Model file for the job. Use its own axes, mm. Face numbers are marked on the shaded views. A direction names the side the tool comes from. Round coordinates to 2 decimals unless told otherwise and drop trailing zeros. Order: outer loops, then holes, each group sorted by start corner. A loop starts at its lowest first (then second) coordinate and runs counter-clockwise, first axis right, second up. Notation, with made-up numbers: (88, -15.75) -> (113, -15.75) arc R25 ccw to (113, 10.25) -> close; hole circle Ø10 at (52, 32.5). An arc over 180 degrees is marked (long way). Put each result on its own line as item: value. Start each with the question number.
Q1. Flat gauge pins, fed straight in: P1, Ø1.5, axis at x = -7.5, z = 2.5, coming from the -Y side; P2, Ø9, axis at x = 0, y = 0, coming from the +Z side; P3, Ø1.5, axis at y = 3, z = 2, coming from the +X side; P4, Ø2, axis at y = 0.5, z = 1, coming from the -X side. Where does each tip first touch, or does it go through?
Q2. Cut at B-B, the plane y = -9. List the corners of the cut face in (x, z), and give its area (3 significant figures).
Q3. Pull direction X, two halves, no side cores. Call the marked faces 5, 6 and 7: released by +X, released by -X, zero draft, split by the parting line, or undercut.
Q4. 3-axis set-ups, long thin cutter, end or side, ignore diameter. For the marked faces 1, 2, 3 and 4: which of +Z, -Z, +X, -X, +Y, -Y reach the whole face in a straight line?
Q5. Probe L1, parallel to Y at x = 0, z = 3.05; L2, parallel to Y at x = -16.5, z = 2.05; L3, parallel to Y at x = 18, z = 3.5. List the from-to ranges inside material, lowest first.
Q6. Cut at A-A, the plane x = 0. List the corners of the cut face in (y, z).
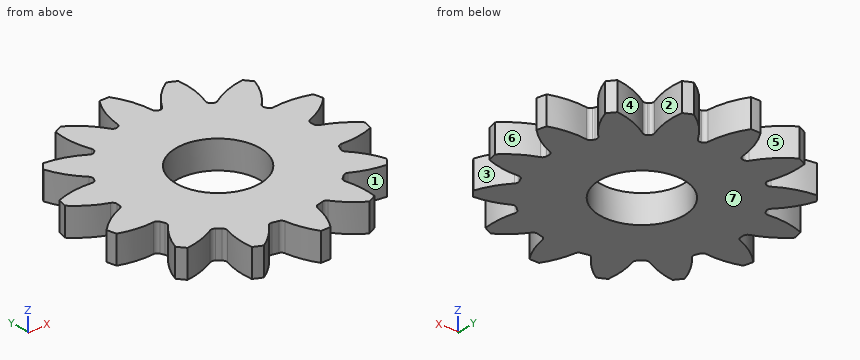
from build123d import *

# Parameters (mm, degrees)
SKETCH_1_R               = 17.25
EXTRUDE_1_DEPTH          = 5
EXTRUDE_2_DEPTH          = 5
FILLET_1_R               = 0.75
PATTERN_CIRCULAR_1_DEPTH = 5
CUT_EXTRUDE_2_REACH      = 35.573
SKETCH_2_R               = 7.5


# Read off the part's stored shape, not the designer's step: 원형 패턴1
with BuildPart() as part:
    # 스케치1 → 보스-돌출1 (new body)
    with BuildSketch(Plane.XY):
        Circle(SKETCH_1_R)
    extrude(amount=EXTRUDE_1_DEPTH)

    # 스케치1<3> → 보스-돌출2 (add)
    with BuildSketch(Plane.XY):
        with BuildLine():
            ThreePointArc((3.105, 16.968249026), (2.435929865, 20.62271117), (0.855, 23.984765477))
            ThreePointArc((0.855, 23.984765477), (0, 24), (-0.855, 23.984765477))
            ThreePointArc((-0.855, 23.984765477), (-2.435929865, 20.62271117), (-3.105, 16.968249026))
            ThreePointArc((-3.105, 16.968249026), (0, 17.25), (3.105, 16.968249026))
        make_face()
    extrude(amount=EXTRUDE_2_DEPTH)

    # 필렛1
    fillet_1_edges = [part.edges().sort_by_distance(p)[0] for p in [
        (-3.105, 16.968249026, 2.5),
        (3.105, 16.968249026, 2.5),
    ]]
    fillet(fillet_1_edges, radius=FILLET_1_R)

    # 원형 패턴1 outline → 원형 패턴1 (add)
    with BuildSketch(Plane.XY):
        with BuildLine():
            ThreePointArc((3.752409392, 16.836921446), (7.228370534, 15.662476159), (10.37732262, 13.77946571))
            ThreePointArc((10.37732262, 13.77946571), (10.109330299, 14.165782518), (10.123973341, 14.635725219))
            ThreePointArc((10.123973341, 14.635725219), (10.902507886, 17.923971687), (10.894078225, 21.303115042))
            ThreePointArc((10.894078225, 21.303115042), (10.130359855, 21.68781147), (9.353421461, 22.045056236))
            ThreePointArc((9.353421461, 22.045056236), (6.66426095, 19.902390957), (4.559090047, 17.183778404))
            ThreePointArc((4.559090047, 17.183778404), (4.211817106, 16.879954744), (3.752409392, 16.836921446))
        make_face()
        with BuildLine():
            ThreePointArc((10.519299619, 13.671387476), (13.161797978, 11.150317215), (15.214303094, 8.129420728))
            ThreePointArc((15.214303094, 8.129420728), (15.133819906, 8.592297997), (15.344497995, 9.012235673))
            ThreePointArc((15.344497995, 9.012235673), (17.375059394, 11.575860868), (18.775450651, 14.531238688))
            ThreePointArc((18.775450651, 14.531238688), (18.2542777, 15.209203175), (17.70928309, 15.868170523))
            ThreePointArc((17.70928309, 15.868170523), (14.414969994, 15.125158945), (11.38395589, 13.636025477))
            ThreePointArc((11.38395589, 13.636025477), (10.94601321, 13.516422059), (10.519299619, 13.671387476))
        make_face()
        with BuildLine():
            ThreePointArc((15.364476978, 7.841896914), (16.663551392, 4.459658622), (17.227504247, 0.880680084))
            ThreePointArc((17.227504247, 0.880680084), (17.349588602, 1.330612703), (17.713914892, 1.62149121))
            ThreePointArc((17.713914892, 1.62149121), (20.511209748, 3.030450816), (22.938114809, 5.010389578))
            ThreePointArc((22.938114809, 5.010389578), (22.762711972, 5.847342943), (22.557604012, 6.677516308))
            ThreePointArc((22.557604012, 6.677516308), (19.379376386, 7.424645609), (16.1145377, 7.437349496))
            ThreePointArc((16.1145377, 7.437349496), (15.676466798, 7.522741397), (15.364476978, 7.841896914))
        make_face()
        with BuildLine():
            ThreePointArc((17.246205523, 0.361794236), (16.948744989, -3.209757512), (15.919681663, -6.642758143))
            ThreePointArc((15.919681663, -6.642758143), (16.218467781, -6.293015235), (16.665227716, -6.183476169))
            ThreePointArc((16.665227716, -6.183476169), (19.653637621, -6.085826774), (22.557604012, -5.373711355))
            ThreePointArc((22.557604012, -5.373711355), (22.762711972, -4.543537991), (22.938114809, -3.706584626))
            ThreePointArc((22.938114809, -3.706584626), (20.519516774, -1.732038623), (17.732464097, -0.324634719))
            ThreePointArc((17.732464097, -0.324634719), (17.384038193, -0.056011184), (17.246205523, 0.361794236))
        make_face()
        with BuildLine():
            ThreePointArc((15.624899975, -7.30924078), (13.802641251, -10.346477396), (11.398453982, -12.947499636))
            ThreePointArc((11.398453982, -12.947499636), (11.812346904, -12.764896736), (12.255961374, -12.853538558))
            ThreePointArc((12.255961374, -12.853538558), (14.896975546, -13.981953909), (17.70928309, -14.56436557))
            ThreePointArc((17.70928309, -14.56436557), (18.2542777, -13.905398222), (18.775450651, -13.227433735))
            ThreePointArc((18.775450651, -13.227433735), (17.528042353, -10.523846266), (15.751756091, -8.13423965))
            ThreePointArc((15.751756091, -8.13423965), (15.562955662, -7.741018123), (15.624899975, -7.30924078))
        make_face()
        with BuildLine():
            ThreePointArc((10.701599161, -13.529163884), (7.742304938, -15.414902343), (4.462626447, -16.662756831))
            ThreePointArc((4.462626447, -16.662756831), (4.907143939, -16.680291261), (5.263531943, -16.946544614))
            ThreePointArc((5.263531943, -16.946544614), (7.123124119, -19.043668749), (9.353421461, -20.741251283))
            ThreePointArc((9.353421461, -20.741251283), (10.130359855, -20.384006517), (10.894078225, -19.99931009))
            ThreePointArc((10.894078225, -19.99931009), (10.952928458, -17.13877644), (10.445613014, -14.322973331))
            ThreePointArc((10.445613014, -14.322973331), (10.45308323, -13.887202628), (10.701599161, -13.529163884))
        make_face()
        with BuildLine():
            ThreePointArc((3.478512175, -16.895634142), (0, -17.25), (-3.478512175, -16.895634142))
            ThreePointArc((-3.478512175, -16.895634142), (-3.093309657, -17.106080205), (-2.891850292, -17.496057961))
            ThreePointArc((-2.891850292, -17.496057961), (-2.126287606, -20.187844374), (-0.855, -22.680960525))
            ThreePointArc((-0.855, -22.680960525), (0, -22.696195047), (0.855, -22.680960525))
            ThreePointArc((0.855, -22.680960525), (2.126287606, -20.187844374), (2.891850292, -17.496057961))
            ThreePointArc((2.891850292, -17.496057961), (3.093309657, -17.106080205), (3.478512175, -16.895634142))
        make_face()
        with BuildLine():
            ThreePointArc((-4.462626447, -16.662756831), (-7.742304938, -15.414902343), (-10.701599161, -13.529163884))
            ThreePointArc((-10.701599161, -13.529163884), (-10.45308323, -13.887202628), (-10.445613014, -14.322973331))
            ThreePointArc((-10.445613014, -14.322973331), (-10.952928458, -17.13877644), (-10.894078225, -19.99931009))
            ThreePointArc((-10.894078225, -19.99931009), (-10.130359855, -20.384006517), (-9.353421461, -20.741251283))
            ThreePointArc((-9.353421461, -20.741251283), (-7.123124119, -19.043668749), (-5.263531943, -16.946544614))
            ThreePointArc((-5.263531943, -16.946544614), (-4.907143939, -16.680291261), (-4.462626447, -16.662756831))
        make_face()
        with BuildLine():
            ThreePointArc((-11.398453982, -12.947499636), (-13.802641251, -10.346477396), (-15.624899975, -7.30924078))
            ThreePointArc((-15.624899975, -7.30924078), (-15.562955662, -7.741018123), (-15.751756091, -8.13423965))
            ThreePointArc((-15.751756091, -8.13423965), (-17.528042353, -10.523846266), (-18.775450651, -13.227433735))
            ThreePointArc((-18.775450651, -13.227433735), (-18.2542777, -13.905398222), (-17.70928309, -14.56436557))
            ThreePointArc((-17.70928309, -14.56436557), (-14.896975546, -13.981953909), (-12.255961374, -12.853538558))
            ThreePointArc((-12.255961374, -12.853538558), (-11.812346904, -12.764896736), (-11.398453982, -12.947499636))
        make_face()
        with BuildLine():
            ThreePointArc((-15.919681663, -6.642758143), (-16.948744989, -3.209757512), (-17.246205523, 0.361794236))
            ThreePointArc((-17.246205523, 0.361794236), (-17.384038193, -0.056011184), (-17.732464097, -0.324634719))
            ThreePointArc((-17.732464097, -0.324634719), (-20.519516774, -1.732038623), (-22.938114809, -3.706584626))
            ThreePointArc((-22.938114809, -3.706584626), (-22.762711972, -4.543537991), (-22.557604012, -5.373711355))
            ThreePointArc((-22.557604012, -5.373711355), (-19.653637621, -6.085826774), (-16.665227716, -6.183476169))
            ThreePointArc((-16.665227716, -6.183476169), (-16.218467781, -6.293015235), (-15.919681663, -6.642758143))
        make_face()
        with BuildLine():
            ThreePointArc((-17.227504247, 0.880680084), (-16.663551392, 4.459658622), (-15.364476978, 7.841896914))
            ThreePointArc((-15.364476978, 7.841896914), (-15.676466798, 7.522741397), (-16.1145377, 7.437349496))
            ThreePointArc((-16.1145377, 7.437349496), (-19.379376386, 7.424645609), (-22.557604012, 6.677516308))
            ThreePointArc((-22.557604012, 6.677516308), (-22.762711972, 5.847342943), (-22.938114809, 5.010389578))
            ThreePointArc((-22.938114809, 5.010389578), (-20.511209748, 3.030450816), (-17.713914892, 1.62149121))
            ThreePointArc((-17.713914892, 1.62149121), (-17.349588602, 1.330612703), (-17.227504247, 0.880680084))
        make_face()
        with BuildLine():
            ThreePointArc((-15.214303094, 8.129420728), (-13.161797978, 11.150317215), (-10.519299619, 13.671387476))
            ThreePointArc((-10.519299619, 13.671387476), (-10.94601321, 13.516422059), (-11.38395589, 13.636025477))
            ThreePointArc((-11.38395589, 13.636025477), (-14.414969994, 15.125158945), (-17.70928309, 15.868170523))
            ThreePointArc((-17.70928309, 15.868170523), (-18.2542777, 15.209203175), (-18.775450651, 14.531238688))
            ThreePointArc((-18.775450651, 14.531238688), (-17.375059394, 11.575860868), (-15.344497995, 9.012235673))
            ThreePointArc((-15.344497995, 9.012235673), (-15.133819906, 8.592297997), (-15.214303094, 8.129420728))
        make_face()
        with BuildLine():
            ThreePointArc((-4.559090047, 17.183778404), (-6.66426095, 19.902390957), (-9.353421461, 22.045056236))
            ThreePointArc((-9.353421461, 22.045056236), (-10.130359855, 21.68781147), (-10.894078225, 21.303115042))
            ThreePointArc((-10.894078225, 21.303115042), (-10.902507886, 17.923971687), (-10.123973341, 14.635725219))
            ThreePointArc((-10.123973341, 14.635725219), (-10.109330299, 14.165782518), (-10.37732262, 13.77946571))
            ThreePointArc((-10.37732262, 13.77946571), (-7.228370534, 15.662476159), (-3.752409392, 16.836921446))
            ThreePointArc((-3.752409392, 16.836921446), (-4.211817106, 16.879954744), (-4.559090047, 17.183778404))
        make_face()
    extrude(amount=PATTERN_CIRCULAR_1_DEPTH)

    # 스케치2 → 컷-돌출2 (cut, up to next)
    with BuildSketch(Plane.XY.offset(5), mode=Mode.PRIVATE) as cut_extrude_2_sk1:
        Circle(SKETCH_2_R)
    cut_extrude_2_tool1 = extrude(cut_extrude_2_sk1.sketch, amount=-CUT_EXTRUDE_2_REACH, mode=Mode.PRIVATE) & part.part
    add(cut_extrude_2_tool1.solids().sort_by_distance((0, 0, 5))[0], mode=Mode.SUBTRACT)


solid = part.part
Ans:
1. P1: stops at y = -19.99
1. P2: passes through
1. P3: stops at x = 21.52
1. P4: stops at x = -18.18
2. outline: (-16.49, 0) -> (16.49, 0) -> (16.49, 5) -> (-16.49, 5) -> close
2. area: 165 mm^2
3. face 5: undercut
3. face 6: released by +X
3. face 7: zero draft
4. face 1: +Z, -Z, -Y
4. face 2: +Z, -Z
4. face 3: +Z, -Z, +X
4. face 4: +Z, -Z, +Y
5. L1: y = -22.7 to -7.5, 7.5 to 24
5. L2: y = -14.39 to -9.02, -6.19 to 7.47, 10.32 to 15.69
5. L3: y = -14.22 to -11.38, -6.22 to -0.43, 1.73 to 7.52, 12.69 to 15.52
6. outline: (-22.7, 0) -> (-7.5, 0) -> (-7.5, 5) -> (-22.7, 5) -> close; (7.5, 0) -> (24, 0) -> (24, 5) -> (7.5, 5) -> close
